from build123d import *

# Parameters (mm, degrees)
SKETCH1_R              = 31.5
ELBOW_PLATE_DEPTH      = 4
SKETCH2_R              = 1.33
HORN_SCREW_HOLES_DEPTH = 4
SKETCH3_R              = 1.33
SCREW_HOLES_DEPTH      = 3
CABLE_SLOT_DEPTH       = 4
FILLET1_R              = 2


with BuildPart() as part:
    # Sketch1 → Elbow Plate (new body)
    with BuildSketch(Plane.XY):
        Circle(SKETCH1_R)
    extrude(amount=ELBOW_PLATE_DEPTH)

    # Sketch2 → Horn Screw Holes (cut)
    with BuildSketch(Plane(origin=(0, 0, 0), x_dir=(-1, 0, 0), z_dir=(0, 0, -1))):
        with Locations((0, 8.25)):
            Circle(SKETCH2_R)
        with Locations((8.25, 0)):
            Circle(SKETCH2_R)
        with Locations((0, -8.25)):
            Circle(SKETCH2_R)
        with Locations((-8.25, 0)):
            Circle(SKETCH2_R)
    extrude(amount=-HORN_SCREW_HOLES_DEPTH, mode=Mode.SUBTRACT)

    # Sketch3 → Screw Holes (cut)
    with BuildSketch(Plane(origin=(0, 0, 0), x_dir=(-1, 0, 0), z_dir=(0, 0, -1))):
        with Locations((22.9496732, 13.25)):
            Circle(SKETCH3_R)
        with Locations((0, 26.5)):
            Circle(SKETCH3_R)
        with Locations((22.9496732, -13.25)):
            Circle(SKETCH3_R)
        with Locations((0, -26.5)):
            Circle(SKETCH3_R)
        with Locations((-22.9496732, -13.25)):
            Circle(SKETCH3_R)
        with Locations((-22.9496732, 13.25)):
            Circle(SKETCH3_R)
    extrude(amount=-SCREW_HOLES_DEPTH, mode=Mode.SUBTRACT)

    # Sketch4 → Cable Slot (cut)
    with BuildSketch(Plane.XY.offset(4)):
        with BuildLine():
            ThreePointArc((0, -23.172318516), (5.001159258, -18.171159258), (0, -13.17))
            ThreePointArc((0, -13.17), (-13.17, 0), (0, 13.17))
            ThreePointArc((0, 13.17), (5.001159258, 18.171159258), (0, 23.172318516))
            ThreePointArc((0, 23.172318516), (-23.172318516, 0), (0, -23.172318516))
        make_face()
    extrude(amount=-CABLE_SLOT_DEPTH, mode=Mode.SUBTRACT)

    # Fillet1
    fillet1_edges = [part.edges().sort_by_distance(p)[0] for p in [
        (-23.172318516, 0, 0),
        (5.001159258, 18.171159258, 0),
        (-13.17, 0, 0),
        (5.001159258, -18.171159258, 0),
    ]]
    fillet(fillet1_edges, radius=FILLET1_R)


solid = part.part
Design review of the part built by this model. Coordinates are the model's own, in mm. A direction names the side the tool comes from. Round coordinates to 2 decimals unless told otherwise and drop trailing zeros. Write each loop counter-clockwise with the first axis right and the second up, starting at its lowest first coordinate (ties: lowest second). Pieces come first, ordered by that corner, then holes.
Item 1: Consider section B-B on z = 1.3. Count the separate pieces of the cut face and the enclosed holes in it, and give its area (3 significant figures).
Item 2: For faces 1 (the cylindrical face through (5, -18, 3)), 2 (the cylindrical face through (-23.56, -14.43, 1.48)), 3 (the flat face through (6.6, 0.4, 4)), list the 3-axis set-ups (+Z, -Z, +X, -X, +Y, -Y) from which the entire face can be reached by the end or side of a thin tool; tool diameter is ignored.
Item 3: Wall thickness on L1, parallel to Y at x = -11.5, z = 3.75; L2, parallel to Z at x = -3, y = -24.5; L3, parallel to X at y = 5.5, z = 0.9: over which ranges is each line inside the solid? List them lowest first.
Item 4: Consider section A-A on y = 0. Give the boundary of the cut face in (x, z), and give its area (3 significant figures).
Item 5: Draft analysis for pull direction X (two halves, no side actions). For faces 4 (the cylindrical face through (6.98, 0.4, 1.97)), 5 (the cylindrical face through (-4.101, 31.232, 1.972)), 6 (the flat face through (6.6, 0.4, 0)), state which applies: released by +X, released by -X, zero draft, split by the parting line, or undercut.
Item 6: Consider section C-C on y = 26.5. Give the boundary of the cut face in (x, z), and give its area (3 significant figures).
Item 7: For pin 1 Ø1.3 at (x, y) = (0, 27) entering from -Z; pin 2 Ø1.5 at (x, z) = (-22.5, 2.5) entering from +Y; pin 3 Ø1.5 at (x, z) = (24.5, 1) entering from -Y, all flat-tipped, find the tip position at first contact; note any pin that passes through.
Check values:
1. separate pieces: 1
1. enclosed holes: 11
1. area: 2,390 mm2
2. face 1: +Z, -Z
2. face 2: -Z
2. face 3: +Z, +X, -X, +Y, -Y
3. L1: y = -29.33 to -20.12, -6.42 to 6.42, 20.12 to 29.33
3. L2: z = 0.06 to 4
3. L3: x = -31.02 to -22.85, -11.6 to 31.02
4. outline: (-31.5, 0) - (-25.17, 0) arc R2 ccw to (-23.17, 2) - (-23.17, 4) - (-31.5, 4) - close; (-13.17, 2) arc R2 ccw to (-11.17, 0) - (-9.58, 0) - (-9.58, 4) - (-13.17, 4) - close; (-6.92, 0) - (6.92, 0) - (6.92, 4) - (-6.92, 4) - close; (9.58, 0) - (31.5, 0) - (31.5, 4) - (9.58, 4) - close
4. area: 189 mm2
5. face 4: undercut
5. face 5: split by the parting line
5. face 6: zero draft
6. outline: (-17.03, 0) - (-1.33, 0) - (-1.33, 3) - (1.33, 3) - (1.33, 0) - (17.03, 0) - (17.03, 4) - (-17.03, 4) - close
6. area: 128 mm2
7. pin 1: stops at z = 3
7. pin 2: stops at y = 22.79
7. pin 3: stops at y = -20.69
